Geometry: see drawing. Coordinates: mm, zero at the bounding-box minimum. A direction names the side the tool comes from. Round coordinates to 2 decimals unless told otherwise and drop trailing zeros. Order: outer loops, then holes, each group sorted by start corner. A loop starts at its lowest first (then second) coordinate and runs counter-clockwise, first axis right, second up. Notation, with made-up numbers: (-23, 38) -> (33, 38) arc R17 cw to (33, 53) -> close; hole circle Ø11 at (47, -30). An arc over 180 degrees is marked (long way). Put each result on its own line as item: value.
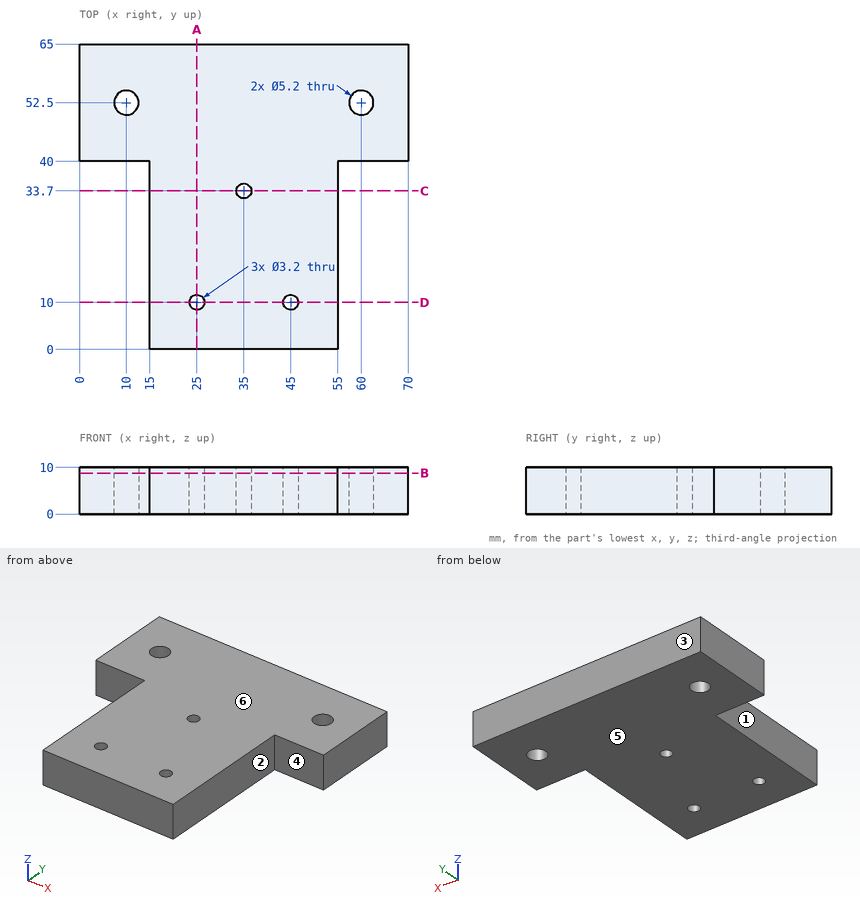
1. Draft query along Z for the marked faces 4, 5 and 6. Return one class per face: +Z half, -Z half, draft (parallel to the pull), parting line (faces both ways), or undercut.
Ans:
face 4: draft
face 5: -Z half
face 6: +Z half
2. Cut plane B-B on z = 8.75. Return loops of the section in (x, y), and give its area (3 significant figures).
Ans:
outline: (0, 40) -> (15, 40) -> (15, 0) -> (55, 0) -> (55, 40) -> (70, 40) -> (70, 65) -> (0, 65) -> close; hole circle Ø5.2 at (10, 52.5); hole circle Ø3.2 at (25, 10); hole circle Ø3.2 at (35, 33.7); hole circle Ø3.2 at (45, 10); hole circle Ø5.2 at (60, 52.5)
area: 3,280 mm²
3. Cut plane C-C on y = 33.7. Return loops of the section in (x, z).
Ans:
outline: (15, 0) -> (33.4, 0) -> (33.4, 10) -> (15, 10) -> close; (36.6, 0) -> (55, 0) -> (55, 10) -> (36.6, 10) -> close
4. Contact query for flat-ended pins moving along their axis: P1, Ø2, axis at y = 33, z = 1.5, coming from the -X side; P2, Ø2.5, axis at x = 25, y = 10, coming from the -Z side; P3, Ø5, axis at x = 24.5, z = 2, coming from the -Y side; P4, Ø3, axis at x = 10, z = 3.5, coming from the -Y side. Output: stop coordinate, or through.
Ans:
P1: x = 15
P2: through
P3: y = 0
P4: y = 40
5. Cut plane A-A on x = 25. Return loops of the section in (y, z).
Ans:
outline: (0, 0) -> (8.4, 0) -> (8.4, 10) -> (0, 10) -> close; (11.6, 0) -> (65, 0) -> (65, 10) -> (11.6, 10) -> close
6. Cut plane D-D on y = 10. Return loops of the section in (x, z), and give its area (3 significant figures).
Ans:
outline: (15, 0) -> (23.4, 0) -> (23.4, 10) -> (15, 10) -> close; (26.6, 0) -> (43.4, 0) -> (43.4, 10) -> (26.6, 10) -> close; (46.6, 0) -> (55, 0) -> (55, 10) -> (46.6, 10) -> close
area: 336 mm²
7. Material intervals for probe 1 along Y at (x, z) = (60, 6.5); probe 2 along Y at (x, z) = (35, 7.5); probe 3 along Y at (x, z) = (56, 9.5), sorted ascending.
Ans:
probe 1: 40 to 49.9, 55.1 to 65
probe 2: 0 to 32.1, 35.3 to 65
probe 3: 40 to 65
8. Set-up query: the marked faces 1, 2 and 3. Return all of +Z, -Z, +X, -X, +Y, -Y with unobstructed straight access to the full face (end or side cutting, diameter ignored); none if empty.
Ans:
face 1: +Z, -Z, -X, -Y
face 2: +Z, -Z, +X, -Y
face 3: +Z, -Z, +X, -X, +Y
